```python
from build123d import *

# Parameters (mm, degrees)
SKETCH1_W           = 14
SKETCH1_H           = 22
SKETCH1_W_2         = 10
SKETCH1_H_2         = 18
EXTRUDE_THIN1_DEPTH = 2
SKETCH2_W           = 2
SKETCH2_H           = 22
BOSS_EXTRUDE1_DEPTH = 4.5
SKETCH3_W           = 22
SKETCH3_H           = 8
SKETCH3_W_2         = 18
SKETCH3_H_2         = 4
EXTRUDE_THIN2_DEPTH = 2
SKETCH4_W           = 20
SKETCH4_H           = 8
CUT_EXTRUDE1_DEPTH  = 26
SKETCH5_W           = 0.9
SKETCH5_H           = 1.9
SKETCH5_H_2         = 3.8
BOSS_EXTRUDE2_DEPTH = 0.9
SKETCH6_W           = 2
SKETCH6_H           = 1.9
BOSS_EXTRUDE3_DEPTH = 8
SKETCH7_W           = 2.8
SKETCH7_H           = 2
BOSS_EXTRUDE4_DEPTH = 0.9
SKETCH8_W           = 0.9
SKETCH8_H           = 0.9
CUT_EXTRUDE2_DEPTH  = 25.657656012
BOSS_EXTRUDE5_REACH = 26.658
SKETCH9_W           = 2
SKETCH9_H           = 3
BOSS_EXTRUDE6_DEPTH = 2
SKETCH11_W          = 1.1
SKETCH11_H          = 3.8
BOSS_EXTRUDE7_DEPTH = 0.9
SKETCH12_W          = 1.1
SKETCH12_H          = 3.8
CUT_EXTRUDE3_DEPTH  = 0.9
FILLET1_R           = 1


with BuildPart() as part:
    # Sketch1 → Extrude-Thin1 (new body)
    with BuildSketch(Plane(origin=(0, 0, 0), x_dir=(1, 0, 0), z_dir=(0, 1, 0))):
        with Locations((5, 9)):
            Rectangle(SKETCH1_W, SKETCH1_H)
        with Locations((5, 9)):
            Rectangle(SKETCH1_W_2, SKETCH1_H_2, mode=Mode.SUBTRACT)
    extrude(amount=EXTRUDE_THIN1_DEPTH)

    # Sketch2 → Boss-Extrude1 (add)
    with BuildSketch(Plane(origin=(0, 2, 0), x_dir=(1, 0, 0), z_dir=(0, 1, 0))):
        with Locations((11, 9)):
            Rectangle(SKETCH2_W, SKETCH2_H)
    extrude(amount=BOSS_EXTRUDE1_DEPTH)

    # Sketch3 → Extrude-Thin2 (add)
    with BuildSketch(Plane.ZY.offset(2)):
        with Locations((-9, 4)):
            Rectangle(SKETCH3_W, SKETCH3_H)
        with Locations((-9, 4)):
            Rectangle(SKETCH3_W_2, SKETCH3_H_2, mode=Mode.SUBTRACT)
    extrude(amount=-EXTRUDE_THIN2_DEPTH)

    # Sketch4 → Cut-Extrude1 (cut)
    with BuildSketch(Plane(origin=(12, 0, 0), x_dir=(0, 0, -1), z_dir=(1, 0, 0))):
        with Locations((8, 4)):
            Rectangle(SKETCH4_W, SKETCH4_H)
    extrude(amount=-CUT_EXTRUDE1_DEPTH, mode=Mode.SUBTRACT)

    # Sketch5 → Boss-Extrude2 (add)
    with BuildSketch(Plane.XY.offset(-18)):
        with Locations((-1.55, 7.05)):
            Rectangle(SKETCH5_W, SKETCH5_H)
        with Locations((-1.55, 0.95)):
            Rectangle(SKETCH5_W, SKETCH5_H)
        with Locations((11.55, 3)):
            Rectangle(SKETCH5_W, SKETCH5_H_2)
    extrude(amount=BOSS_EXTRUDE2_DEPTH)

    # Sketch6 → Boss-Extrude3 (add)
    with BuildSketch(Plane.ZY.offset(2)):
        Polygon((-18, 1.9), (-18, 6.1), (-18, 8), (-20, 8), (-20, 1.9), align=None)
        with Locations((-19, 0.95)):
            Rectangle(SKETCH6_W, SKETCH6_H)
    extrude(amount=BOSS_EXTRUDE3_DEPTH)

    # Sketch7 → Boss-Extrude4 (add)
    with BuildSketch(Plane.XY.offset(-18)):
        with Locations((-5, 7)):
            Rectangle(SKETCH7_W, SKETCH7_H)
        with Locations((-5, 1)):
            Rectangle(SKETCH7_W, SKETCH7_H)
    extrude(amount=BOSS_EXTRUDE4_DEPTH)

    # Sketch8 → Cut-Extrude2 (cut, through all)
    with BuildSketch(Plane(origin=(0, 8, 0), x_dir=(1, 0, 0), z_dir=(0, 1, 0))):
        with Locations((-1.55, 17.55)):
            Rectangle(SKETCH8_W, SKETCH8_H)
    extrude(amount=-CUT_EXTRUDE2_DEPTH, mode=Mode.SUBTRACT)

    # Sketch9 → Boss-Extrude5 (add, up to next)
    with BuildSketch(Plane(origin=(0, 0, 0), x_dir=(0, 0, -1), z_dir=(1, 0, 0)), mode=Mode.PRIVATE) as boss_extrude5_sk1:
        with Locations((19, 3.5)):
            Rectangle(SKETCH9_W, SKETCH9_H)
    boss_extrude5_tool1 = extrude(boss_extrude5_sk1.sketch, amount=BOSS_EXTRUDE5_REACH, mode=Mode.PRIVATE) - part.part
    add(boss_extrude5_tool1.solids().sort_by_distance((0, 3.5, -19))[0])

    # Sketch10 → Boss-Extrude6 (add)
    with BuildSketch(Plane(origin=(12, 0, 0), x_dir=(0, 0, -1), z_dir=(1, 0, 0))):
        Polygon((18, 6.5), (18, 4.9), (17.1, 4.9), (17.1, 1.1), (18, 1.1), (18, 0), (20, 0), (20, 6.5), align=None)
    extrude(amount=BOSS_EXTRUDE6_DEPTH)

    # Sketch11 → Boss-Extrude7 (add)
    with BuildSketch(Plane.XY.offset(-18)):
        with Locations((10.55, 3)):
            Rectangle(SKETCH11_W, SKETCH11_H)
    extrude(amount=BOSS_EXTRUDE7_DEPTH)

    # Sketch12 → Cut-Extrude3 (cut)
    with BuildSketch(Plane.XY.offset(-17.1)):
        with Locations((10.55, 3)):
            Rectangle(SKETCH12_W, SKETCH12_H)
        with Locations((13.45, 3)):
            Rectangle(SKETCH12_W, SKETCH12_H)
    extrude(amount=-CUT_EXTRUDE3_DEPTH, mode=Mode.SUBTRACT)

    # Fillet1
    fillet1_edges = [part.edges().sort_by_distance(p)[0] for p in [
        (-10, 0, -19),
        (-10, 8, -19),
        (14, 6.5, -19),
        (14, 0, -19),
        (10, 6.5, -19),
        (0, 8, -19),
    ]]
    fillet(fillet1_edges, radius=FILLET1_R)


solid = part.part
```
Can you work these out from the model? Positions are in its coordinate system, mm. A direction names the side the tool comes from. Coordinates: 2 decimals unless noted, no trailing zeros. Loops run counter-clockwise (first coordinate to the right, second up) from the corner with the lowest first, then second, coordinate; pieces in that order, holes last.
Item 1: Suppose I cut it at B-B (y = 5.75). Please give me the cut outline in (x, z), then the cut area to 3 significant figures.
Answers below:
outline: (-10, -20) - (0, -20) - (0, -18) - (-10, -18) - close; (10.03, -20) - (13.97, -20) - (13.97, -18) - (10.03, -18) - close
area: 27.9 mm2
Item 2: I'm going to push flat-ended pins straight in: pin 1 (0.7 mm diameter, centred on x = 12.5, z = -17.5, fed in from -Y); pin 2 (0.7 mm diameter, centred on y = 1, z = -17.5, fed in from +X); pin 3 (1 mm diameter, centred on x = -2, y = 5.5, fed in from +Z). Where does each tip first touch, or does it pass through?
Answers below:
pin 1: stops at y = 1.1
pin 2: stops at x = 12.9
pin 3: stops at z = -18
Item 3: Suppose I cut it at A-A (z = -17.75). Please give me the cut outline in (x, y).
Answers below:
outline: (-6.4, 0) - (-3.6, 0) - (-3.6, 2) - (-6.4, 2) - close; (-6.4, 6) - (-3.6, 6) - (-3.6, 8) - (-6.4, 8) - close; (11.1, 1.1) - (12.9, 1.1) - (12.9, 4.9) - (11.1, 4.9) - close
Item 4: Please list where these lines run through material, in increasing order: L1, parallel to X at y = 5.5, z = -19.25; L2, parallel to X at y = 6.5, z = -17.4; L3, parallel to Z at x = -8, y = 4.75.
Answers below:
L1: x = -10 to 0, 10 to 14
L2: x = -6.4 to -3.6
L3: z = -20 to -18
Item 5: Suppose I cut it at C-C (x = -6). Please give me the cut outline in (y, z).
Answers below:
outline: (0, -20) - (8, -20) - (8, -17.1) - (6, -17.1) - (6, -18) - (2, -18) - (2, -17.1) - (0, -17.1) - close
Item 6: Suppose I cut it at D-D (z = -19). Please give me the cut outline in (x, y), then the cut area to 3 significant figures.
Answers below:
outline: (-10, 1) arc R1 ccw to (-9, 0) - (13, 0) arc R1 ccw to (14, 1) - (14, 5.5) arc R1 ccw to (13, 6.5) - (11, 6.5) arc R1 ccw to (10, 5.5) - (10, 5) - (0, 5) - (0, 7) arc R1 ccw to (-1, 8) - (-9, 8) arc R1 ccw to (-10, 7) - close
area: 155 mm2
Item 7: If we mould it in two halves opening along Y, with no side actions, what happens to faces 6 (the face through (14, 3, -19)), 7 (the face through (-5, 2, -17.6)), 8 (the face through (2, 0, -19)), 9 (the face through (13.715, 6.199, -18.986))? For each: released by +Y, released by -Y, zero draft, split by the parting line, or undercut.
Answers below:
face 6: zero draft
face 7: undercut
face 8: released by -Y
face 9: released by +Y
Item 8: Which directions (+Z, -Z, +X, -X, +Y, -Y) give clear straight access to the entire face, cutting with the end or side of a thin tool? Please do faces 1 (the face through (12, 6.5, -19)), 2 (the face through (5, 5, -19)), 3 (the face through (-3.6, 7, -17.6)), 4 (the face through (-6.4, 7, -17.6)), 5 (the face through (-5, 6, -17.6)).
Answers below:
face 1: +Z, -Z, +X, +Y
face 2: +Z, -Z, +Y
face 3: +Z, +X, +Y, -Y
face 4: +Z, -X, +Y, -Y
face 5: +Z, +X, -X
